For this review, take the finished solid that the model builds, in its own axes (mm). A direction names the side the tool comes from. Give positions to 0.01 mm unless a question says otherwise; leave off trailing zeros. Order: outer loops, then holes, each group sorted by start corner. A loop starts at its lowest first (then second) coordinate and runs counter-clockwise, first axis right, second up. Notation, with made-up numbers: (7, 84.5) - (56, 84.5) arc R3 cw to (56, 88.5) - close; hole circle Ø7 at (-13, -12). An arc over 180 degrees is marked (long way). Use a Markdown table: item, result. Add a question column.
1) We need section D-D on x = 28.5. Write out the cut boundary in (y, z), then the cut area to 3 significant figures.
2) Clearance check with flat-ended pins moving along their axes: P1, Ø2, axis at x = 14.5, z = -12, coming from the -Y side; P2, Ø6.5, axis at y = 24.5, z = -9.5, coming from the -X side; P3, Ø5, axis at x = 24.5, z = -2.5, coming from the +Y side. State where each tip first meets the part, or that it passes through.
3) Machinability: for faces 5 (the face through (20.376, -10.479, -14.053)), 6 (the face through (0.99, 27.63, -14.56)), 7 (the face through (24, -9, -10)), 8 (the face through (23, -14, -12)), which of the approach directions +Z, -Z, +X, -X, +Y, -Y give a long, thin tool a straight path to every point of the face, cutting with its end or side? Answer none if there is none.
4) Mouldability with a two-part tool opening along Z and no side actions: class faces 1 (the face through (2, 33, -10)), 2 (the face through (15, -12, -9)), 3 (the face through (7, 3, -10)), 4 (the face through (14.914, -13.014, -9.675)) as released by +Z, released by -Z, zero draft, split by the parting line, or undercut.
5) We need section B-B on x = 20.5. Write out the cut boundary in (y, z), then the cut area to 3 significant figures.
6) We need section A-A on y = -2.5. Write out the cut boundary in (x, z), then the cut area to 3 significant figures.
7) Wall thickness on L1, parallel to Y at x = 4.15, z = -10; L2, parallel to X at y = -10.95, z = -10; L3, parallel to X at y = -7.5, z = -7.75: over which ranges is each line inside the solid? List them lowest first.
```python
from build123d import *

# Parameters (mm, degrees)
SKETCH1_W                = 41
SKETCH1_H                = 20
BOSS_EXTRUDE2_DEPTH      = 7
SKETCH3_R                = 10.05
CUT_EXTRUDE8_DEPTH       = 2
SKETCH4_R                = 1.5
SKETCH4_R_2              = 3
CUT_EXTRUDE9_DEPTH       = 29
SKETCH5_W                = 6
SKETCH5_H                = 20
SKETCH5_W_2              = 7
BOSS_EXTRUDE3_DEPTH      = 36
CUT_EXTRUDE10_DEPTH      = 36
SKETCH7_R                = 2
CUT_EXTRUDE11_DEPTH      = 51
SKETCH8_R                = 10.05
CUT_EXTRUDE12_DEPTH      = 2
SKETCH9_R                = 4.75
CUT_EXTRUDE13_DEPTH      = 3.25
SKETCH10_R               = 6.5
CUT_EXTRUDE14_DEPTH      = 2
CUT_EXTRUDE15_DEPTH      = 14
CUT_EXTRUDE15_DEPTH_BACK = 10
SKETCH12_R               = 1.5
CUT_EXTRUDE16_DEPTH      = 10
CUT_EXTRUDE17_DEPTH      = 10
MIRROR1_START            = 5
MIRROR1_DEPTH            = 2
MIRROR1_2_DEPTH          = 7
MIRROR1_3_DEPTH          = 5
CUT_EXTRUDE18_DEPTH      = 10
CUT_EXTRUDE18_DEPTH_BACK = 10
BOSS_EXTRUDE4_START      = 16
BOSS_EXTRUDE4_DEPTH      = 16
BOSS_EXTRUDE6_START      = -21
SKETCH16_W               = 28
SKETCH16_H               = 20
SKETCH16_R               = 1.5
SKETCH16_R_2             = 3
BOSS_EXTRUDE6_DEPTH      = 21
SKETCH18_W               = 28
SKETCH18_H               = 20
CUT_EXTRUDE21_DEPTH      = 16
CROQUIS2_R               = 3
CORTAR_EXTRUIR1_DEPTH    = 3
CROQUIS3_R               = 4
CORTAR_EXTRUIR2_DEPTH    = 0.3


# Read off the part's stored shape, not the designer's step: Mirror1
with BuildPart() as part:
    # Sketch1 → Boss-Extrude2 (new body)
    with BuildSketch(Plane(origin=(0, 0, 0), x_dir=(1, 0, 0), z_dir=(0, 1, 0))):
        with Locations((20.5, 10)):
            Rectangle(SKETCH1_W, SKETCH1_H)
    extrude(amount=BOSS_EXTRUDE2_DEPTH)

    # Sketch3 → Cut-Extrude8 (cut)
    with BuildSketch(Plane.XZ):
        with Locations((20.5, -10)):
            Circle(SKETCH3_R)
    extrude(amount=-CUT_EXTRUDE8_DEPTH, mode=Mode.SUBTRACT)

    # Sketch4 → Cut-Extrude9 (cut)
    with BuildSketch(Plane.XZ.offset(-2)):
        with Locations(Location((20.5, -2.95, 0), (0, 0, 270))):
            Circle(SKETCH4_R)
        with Locations(Location((27.55, -10, 0), (0, 0, 270))):
            Circle(SKETCH4_R)
        with Locations(Location((20.5, -17.05, 0), (0, 0, 270))):
            Circle(SKETCH4_R)
        with Locations(Location((13.45, -10, 0), (0, 0, 270))):
            Circle(SKETCH4_R)
        with Locations(Location((20.5, -10, 0), (0, 0, 270))):
            Circle(SKETCH4_R_2)
    extrude(amount=-CUT_EXTRUDE9_DEPTH, mode=Mode.SUBTRACT)

    # Sketch5 → Boss-Extrude3 (add)
    with BuildSketch(Plane(origin=(0, 7, 0), x_dir=(1, 0, 0), z_dir=(0, 1, 0))):
        with Locations((38, 10)):
            Rectangle(SKETCH5_W, SKETCH5_H)
        with Locations((3.5, 10)):
            Rectangle(SKETCH5_W_2, SKETCH5_H)
    extrude(amount=BOSS_EXTRUDE3_DEPTH)

    # Sketch6 → Cut-Extrude10 (cut)
    with BuildSketch(Plane.XY):
        Polygon((0, 33), (71.43253461, 33), (71.43253461, 55.308458538), (-13.966778087, 55.308458538), align=None)
    extrude(amount=-CUT_EXTRUDE10_DEPTH, mode=Mode.SUBTRACT)

    # Sketch7 → Cut-Extrude11 (cut)
    with BuildSketch(Plane.ZY):
        with Locations((-10, 23)):
            Circle(SKETCH7_R)
    extrude(amount=-CUT_EXTRUDE11_DEPTH, mode=Mode.SUBTRACT)

    # Sketch8 → Cut-Extrude12 (cut)
    with BuildSketch(Plane.ZY):
        with Locations((-10, 23)):
            Circle(SKETCH8_R)
    extrude(amount=-CUT_EXTRUDE12_DEPTH, mode=Mode.SUBTRACT)

    # Sketch9 → Cut-Extrude13 (cut)
    with BuildSketch(Plane.ZY.offset(-2)):
        with Locations((-10, 23)):
            Circle(SKETCH9_R)
    extrude(amount=-CUT_EXTRUDE13_DEPTH, mode=Mode.SUBTRACT)

    # Sketch10 → Cut-Extrude14 (cut)
    with BuildSketch(Plane(origin=(7, 0, 0), x_dir=(0, 0, -1), z_dir=(1, 0, 0))):
        with Locations((10, 23)):
            Circle(SKETCH10_R)
    extrude(amount=-CUT_EXTRUDE14_DEPTH, mode=Mode.SUBTRACT)

    # Sketch11 → Cut-Extrude15 (cut, two sides: drawn at the far end of the back side and taken through both)
    with BuildSketch(Plane.ZY.offset(-2).offset(-CUT_EXTRUDE15_DEPTH_BACK)):
        with BuildLine():
            Line((0, 23), (15.490351621, 23))
            Line((15.490351621, 23), (12.295560885, 45.157965149))
            Line((12.295560885, 45.157965149), (-24.464924867, 45.157965149))
            Line((-24.464924867, 45.157965149), (-29.902866546, 24.493786768))
            Line((-29.902866546, 24.493786768), (-20, 23))
            ThreePointArc((-20, 23), (-10, 33), (0, 23))
        make_face()
    extrude(amount=CUT_EXTRUDE15_DEPTH + CUT_EXTRUDE15_DEPTH_BACK, mode=Mode.SUBTRACT)

    # Sketch12 → Cut-Extrude16 (cut)
    with BuildSketch(Plane.ZY.offset(-2)):
        with Locations((-10, 30)):
            Circle(SKETCH12_R)
        with Locations((-3, 23)):
            Circle(SKETCH12_R)
        with Locations((-10, 16)):
            Circle(SKETCH12_R)
        with Locations((-17, 23)):
            Circle(SKETCH12_R)
    extrude(amount=-CUT_EXTRUDE16_DEPTH, mode=Mode.SUBTRACT)

    # Sketch13 → Cut-Extrude17 (cut)
    with BuildSketch(Plane(origin=(41, 0, 0), x_dir=(0, 0, -1), z_dir=(1, 0, 0))):
        with BuildLine():
            Line((20, 23), (26.17535893, 23))
            Line((26.17535893, 23), (24.098367316, 34.532076054))
            Line((24.098367316, 34.532076054), (-4.476002155, 34.532076054))
            Line((-4.476002155, 34.532076054), (-5.608906672, 23))
            Line((-5.608906672, 23), (0, 23))
            ThreePointArc((0, 23), (10, 33), (20, 23))
        make_face()
    extrude(amount=-CUT_EXTRUDE17_DEPTH, mode=Mode.SUBTRACT)

    # Mirror1 outline → Mirror1 (cut)
    with BuildSketch(Plane.YZ.offset(MIRROR1_START)):
        with BuildLine():
            Line((23, 0), (21.99875078, 0))
            ThreePointArc((21.99875078, 0), (12.95, -10), (21.99875078, -20))
            Line((21.99875078, -20), (23, -20))
            ThreePointArc((23, -20), (33, -10), (23, 0))
        make_face()
        with BuildLine():
            ThreePointArc((24.355261854, -16.357142857), (23, -18.5), (21.644738146, -16.357142857))
            ThreePointArc((21.644738146, -16.357142857), (18.403805922, -14.596194078), (16.642857143, -11.355261854))
            ThreePointArc((16.642857143, -11.355261854), (14.5, -10), (16.642857143, -8.644738146))
            ThreePointArc((16.642857143, -8.644738146), (18.403805922, -5.403805922), (21.644738146, -3.642857143))
            ThreePointArc((21.644738146, -3.642857143), (23, -1.5), (24.355261854, -3.642857143))
            ThreePointArc((24.355261854, -3.642857143), (27.596194078, -5.403805922), (29.357142857, -8.644738146))
            ThreePointArc((29.357142857, -8.644738146), (31.5, -10), (29.357142857, -11.355261854))
            ThreePointArc((29.357142857, -11.355261854), (27.596194078, -14.596194078), (24.355261854, -16.357142857))
        make_face(mode=Mode.SUBTRACT)
    extrude(amount=MIRROR1_DEPTH, mode=Mode.SUBTRACT)



with BuildPart() as body_2:
    # Mirror1 2 outline → Mirror1 2 (new body)
    with BuildSketch(Plane.YZ):
        with BuildLine():
            Line((43, 0), (24.00124922, 0))
            ThreePointArc((24.00124922, 0), (33.05, -10), (24.00124922, -20))
            Line((24.00124922, -20), (43, -20))
            Line((43, -20), (43, 0))
        make_face()
    extrude(amount=MIRROR1_2_DEPTH)


with BuildPart() as part_1:
    add(part.part)

    add(body_2.part)  # Mirror1 3 merges body 2
    # Mirror1 3 outline → Mirror1 3 (add)
    with BuildSketch(Plane.YZ):
        with BuildLine():
            ThreePointArc((21.99875078, 0), (12.95, -10), (21.99875078, -20))
            Line((21.99875078, -20), (24.00124922, -20))
            ThreePointArc((24.00124922, -20), (33.05, -10), (24.00124922, 0))
            Line((24.00124922, 0), (21.99875078, 0))
        make_face()
        with BuildLine():
            ThreePointArc((24.355261854, -16.357142857), (23, -18.5), (21.644738146, -16.357142857))
            ThreePointArc((21.644738146, -16.357142857), (18.403805922, -14.596194078), (16.642857143, -11.355261854))
            ThreePointArc((16.642857143, -11.355261854), (14.5, -10), (16.642857143, -8.644738146))
            ThreePointArc((16.642857143, -8.644738146), (18.403805922, -5.403805922), (21.644738146, -3.642857143))
            ThreePointArc((21.644738146, -3.642857143), (23, -1.5), (24.355261854, -3.642857143))
            ThreePointArc((24.355261854, -3.642857143), (27.596194078, -5.403805922), (29.357142857, -8.644738146))
            ThreePointArc((29.357142857, -8.644738146), (31.5, -10), (29.357142857, -11.355261854))
            ThreePointArc((29.357142857, -11.355261854), (27.596194078, -14.596194078), (24.355261854, -16.357142857))
        make_face(mode=Mode.SUBTRACT)
    extrude(amount=MIRROR1_3_DEPTH)

    # Sketch14 → Cut-Extrude18 (cut, two sides: drawn at the far end of the back side and taken through both)
    with BuildSketch(Plane(origin=(5, 0, 0), x_dir=(0, 0, -1), z_dir=(1, 0, 0)).offset(-CUT_EXTRUDE18_DEPTH_BACK)):
        with BuildLine():
            Line((20, 23), (39.442144398, 23))
            Line((39.442144398, 23), (24.053498228, 52.618460363))
            Line((24.053498228, 52.618460363), (-15.863160605, 48.721271778))
            Line((-15.863160605, 48.721271778), (-25.901373625, 22.149531431))
            Line((-25.901373625, 22.149531431), (0, 23))
            ThreePointArc((0, 23), (10, 33), (20, 23))
        make_face()
    extrude(amount=CUT_EXTRUDE18_DEPTH + CUT_EXTRUDE18_DEPTH_BACK, mode=Mode.SUBTRACT)

    # Sketch15 → Boss-Extrude4 (add)
    with BuildSketch(Plane.XZ.offset(BOSS_EXTRUDE4_START)):
        with BuildLine():
            Line((21.50124922, 0), (41, 0))
            Line((41, 0), (41, -20))
            Line((41, -20), (21.50124922, -20))
            ThreePointArc((21.50124922, -20), (30.55, -10), (21.50124922, 0))
        make_face()
        with BuildLine():
            Line((0, 0), (19.49875078, 0))
            ThreePointArc((19.49875078, 0), (10.45, -10), (19.49875078, -20))
            Line((19.49875078, -20), (0, -20))
            Line((0, -20), (0, 0))
        make_face()
    extrude(amount=-BOSS_EXTRUDE4_DEPTH)

    # Sketch16 → Boss-Extrude6 (add)
    with BuildSketch(Plane(origin=(0, 7, 0), x_dir=(1, 0, 0), z_dir=(0, 1, 0)).offset(BOSS_EXTRUDE6_START)):
        with Locations((21, 10)):
            Rectangle(SKETCH16_W, SKETCH16_H)
        with Locations(Location((27.55, 10, 0), (0, 0, 90))):
            Circle(SKETCH16_R, mode=Mode.SUBTRACT)
        with Locations(Location((20.5, 10, 0), (0, 0, 90))):
            Circle(SKETCH16_R_2, mode=Mode.SUBTRACT)
        with Locations(Location((13.45, 10, 0), (0, 0, 90))):
            Circle(SKETCH16_R, mode=Mode.SUBTRACT)
        with Locations(Location((20.5, 17.05, 0), (0, 0, 90))):
            Circle(SKETCH16_R, mode=Mode.SUBTRACT)
        with Locations(Location((20.5, 2.95, 0), (0, 0, 90))):
            Circle(SKETCH16_R, mode=Mode.SUBTRACT)
    extrude(amount=BOSS_EXTRUDE6_DEPTH)

    # Sketch18 → Cut-Extrude21 (cut)
    with BuildSketch(Plane(origin=(0, 7, 0), x_dir=(1, 0, 0), z_dir=(0, 1, 0))):
        with Locations((21, 10)):
            Rectangle(SKETCH18_W, SKETCH18_H)
    extrude(amount=-CUT_EXTRUDE21_DEPTH, mode=Mode.SUBTRACT)

    # Croquis2 → Cortar-Extruir1 (cut)
    with BuildSketch(Plane(origin=(0, -9, 0), x_dir=(1, 0, 0), z_dir=(0, 1, 0))):
        with Locations(Location((27.55, 10, 0), (0, 0, 270))):
            Circle(CROQUIS2_R)
        with Locations((20.5, 17.05)):
            Circle(CROQUIS2_R)
        with Locations(Location((13.45, 10, 0), (0, 0, 270))):
            Circle(CROQUIS2_R)
        with Locations((20.5, 2.95)):
            Circle(CROQUIS2_R)
    extrude(amount=-CORTAR_EXTRUIR1_DEPTH, mode=Mode.SUBTRACT)

    # Croquis3 → Cortar-Extruir2 (cut)
    with BuildSketch(Plane.ZY.offset(-35)):
        with Locations((-10, 23)):
            Circle(CROQUIS3_R)
    extrude(amount=-CORTAR_EXTRUIR2_DEPTH, mode=Mode.SUBTRACT)


solid = part_1.part
```
Checked values:
| question | item | result |
|---|---|---|
| 1 | outline | (-16, -20) - (-9, -20) - (-9, -12.85) - (-12, -12.85) - (-12, -11.16) - (-14, -11.16) - (-14, -16.08) - (-16, -16.08) - close; (-16, -3.92) - (-14, -3.92) - (-14, -8.84) - (-12, -8.84) - (-12, -7.15) - (-9, -7.15) - (-9, 0) - (-16, 0) - close |
| 1 | area | 94.0 mm² |
| 2 | P1 | y = -14 |
| 2 | P2 | x = 2 |
| 2 | P3 | y = -9 |
| 3 | face 5 | +Y |
| 3 | face 6 | -X |
| 3 | face 7 | +Z, -Z, +Y |
| 3 | face 8 | -Y |
| 4 | face 1 | split by the parting line |
| 4 | face 2 | undercut |
| 4 | face 3 | zero draft |
| 4 | face 4 | undercut |
| 5 | outline | (-14, -20) - (-12, -20) - (-12, -18.55) - (-14, -18.55) - close; (-14, -15.55) - (-12, -15.55) - (-12, -14.05) - (-9, -14.05) - (-9, -13) - (-14, -13) - close; (-14, -7) - (-9, -7) - (-9, -5.95) - (-12, -5.95) - (-12, -4.45) - (-14, -4.45) - close; (-14, -1.45) - (-12, -1.45) - (-12, 0) - (-14, 0) - close |
| 5 | area | 22.3 mm² |
| 6 | outline | (0, -20) - (7, -20) - (7, 0) - (0, 0) - close; (35, -20) - (41, -20) - (41, 0) - (35, 0) - close |
| 6 | area | 260 mm² |
| 7 | L1 | -16 to 14.5, 17.5 to 18.25, 27.75 to 28.5, 31.5 to 33 |
| 7 | L2 | 0 to 10.45, 16.45 to 17.5, 23.5 to 24.55, 30.55 to 41 |
| 7 | L3 | 0 to 7, 35 to 41 |
